Here's how the part is built. I have some questions about the finished solid (model axes, mm). A direction names the side the tool comes from. Give positions to 0.01 mm unless a question says otherwise; leave off trailing zeros. Loops run counter-clockwise (first coordinate to the right, second up) from the corner with the lowest first, then second, coordinate; pieces in that order, holes last. Notation, with made-up numbers: (33, -34.75) - (71, -34.75) arc R19 ccw to (71, -10.75) - close; hole circle Ø9 at (70.25, -29). An arc over 180 degrees is marked (long way). One line per item, written item: value. Start each with the question number.
```python
from build123d import *

# Parameters (mm, degrees)
SKETCH_1_W          = 32
SKETCH_1_H          = 23
EXTRUDE_1_DEPTH     = 2
SKETCH_4_R          = 2.5
EXTRUDE_2_DEPTH     = 5
SKETCH_5_R          = 1
CUT_EXTRUDE_1_DEPTH = 8
SKETCH_7_R          = 2
CUT_EXTRUDE_2_DEPTH = 3
FILLET_1_R          = 2
FILLET_2_R          = 2
FILLET_3_R          = 2
FILLET_4_R          = 2


with BuildPart() as part:
    # Эскиз1 → Бобышка-Вытянуть1 (new body)
    with BuildSketch(Plane(origin=(0, 0, 0), x_dir=(1, 0, 0), z_dir=(0, 1, 0))):
        with Locations((16, -11.5)):
            Rectangle(SKETCH_1_W, SKETCH_1_H)
    extrude(amount=EXTRUDE_1_DEPTH)

    # Эскиз4 → Бобышка-Вытянуть2 (add)
    with BuildSketch(Plane(origin=(0, 2, 0), x_dir=(1, 0, 0), z_dir=(0, 1, 0))):
        with Locations((18, -8)):
            Circle(SKETCH_4_R)
        with Locations((6.5, -15)):
            Circle(SKETCH_4_R)
    extrude(amount=EXTRUDE_2_DEPTH)

    # Эскиз5 → Вырез-Вытянуть1 (cut, through all)
    with BuildSketch(Plane(origin=(0, 7, 0), x_dir=(1, 0, 0), z_dir=(0, 1, 0))):
        with Locations((6.5, -15)):
            Circle(SKETCH_5_R)
        with Locations((18, -8)):
            Circle(SKETCH_5_R)
    extrude(amount=-CUT_EXTRUDE_1_DEPTH, mode=Mode.SUBTRACT)

    # Эскиз7 → Вырез-Вытянуть2 (cut, through all)
    with BuildSketch(Plane(origin=(0, 2, 0), x_dir=(1, 0, 0), z_dir=(0, 1, 0))):
        with Locations((7, -3)):
            Circle(SKETCH_7_R)
        with Locations((20, -20)):
            Circle(SKETCH_7_R)
    extrude(amount=-CUT_EXTRUDE_2_DEPTH, mode=Mode.SUBTRACT)

    # Скругление1
    fillet_1_edges = [part.edges().sort_by_distance(p)[0] for p in [
        (0, 1, 0),
    ]]
    fillet(fillet_1_edges, radius=FILLET_1_R)

    # Скругление2
    fillet_2_edges = [part.edges().sort_by_distance(p)[0] for p in [
        (0, 1, 23),
    ]]
    fillet(fillet_2_edges, radius=FILLET_2_R)

    # Скругление3
    fillet_3_edges = [part.edges().sort_by_distance(p)[0] for p in [
        (32, 1, 23),
    ]]
    fillet(fillet_3_edges, radius=FILLET_3_R)

    # Скругление4
    fillet_4_edges = [part.edges().sort_by_distance(p)[0] for p in [
        (32, 1, 0),
    ]]
    fillet(fillet_4_edges, radius=FILLET_4_R)


solid = part.part
```
(1) If we section it at A-A on x = 20: List the corners of the cut face in (y, z) for me.
(2) If we section it at D-D on z = 3: List the corners of the cut face in (x, y) for me, plus the area to 3 significant figures.
(3) If we section it at C-C on y = 4: List the corners of the cut face in (x, z) for me.
(4) Will these pins go through, and if not, where does the flat tip stop? pin 1 (2.5 mm diameter, centred on x = 20, z = 20, fed in from +Y); pin 2 (1 mm diameter, centred on x = 6, y = 4, fed in from +Z).
(5) For faces 1 (the face through (8.81, 4.46, 15.96)), 2 (the face through (0.57, 1.01, 0.6)), which set-ups out of +Z, -Z, +X, -X, +Y, -Y let a thin tool reach every point of the face, with its end or its side?
(6) Please list where these lines run through material, in increasing order: probe 1 along X at (y, z) = (4, 15); probe 2 along Z at (x, y) = (18, 4.5); probe 3 along X at (y, z) = (2.5, 8). Write a range as from..to.
(7) If we mould it in two halves opening along X, with no side actions, what happens to faces 3 (the face through (5.4, 1, 4.2)), 4 (the face through (16, 4.5, 9.5)), 5 (the face through (16, 2, 11))? For each: pulls with the +X half, pulls with the -X half, needs draft (parallel to the pull), parting line crosses it, or undercut.
(8) If we section it at B-B on z = 15: List the corners of the cut face in (x, y) for me, plus the area to 3 significant figures.
Found:
1. outline: (0, 0) - (2, 0) - (2, 6.5) - (7, 6.5) - (7, 9.5) - (2, 9.5) - (2, 18) - (0, 18) - close; (0, 22) - (2, 22) - (2, 23) - (0, 23) - close
2. outline: (0, 0) - (5, 0) - (5, 2) - (0, 2) - close; (9, 0) - (32, 0) - (32, 2) - (9, 2) - close
2. area: 56.0 mm^2
3. outline: circle Ø5 at (6.5, 15); circle Ø5 at (18, 8); hole circle Ø2 at (6.5, 15); hole circle Ø2 at (18, 8)
4. pin 1: through
4. pin 2: z = 17.5
5. face 1: +Y
5. face 2: -Z, -X, +Y, -Y
6. probe 1: 4..5.5, 7.5..9
6. probe 2: 5.5..7, 9..10.5
6. probe 3: 15.5..17, 19..20.5
7. face 3: undercut
7. face 4: parting line crosses it
7. face 5: needs draft
8. outline: (0, 0) - (5.5, 0) - (5.5, 7) - (4, 7) - (4, 2) - (0, 2) - close; (7.5, 0) - (32, 0) - (32, 2) - (9, 2) - (9, 7) - (7.5, 7) - close
8. area: 75.0 mm^2
